Input: part model. Units: mm. Frame: model coordinates. Face numbers are marked on the shaded views. Round coordinates to 2 decimals unless told otherwise and drop trailing zeros. Loops run counter-clockwise (first coordinate to the right, second up) from the corner with the lowest first, then second, coordinate; pieces in that order, holes last.
1) Section B-B, the plane x = -1.6. Return loops of the section in (y, z), and give its area (3 significant figures).
2) Draft query along Z for the marked faces 1, 2, 3 and 4. Return one class per face: pulls with the +Z half, pulls with the -Z half, needs draft (parallel to the pull), parting line crosses it, or undercut.
3) First-contact query: pin 1 (1.5 mm diameter, centred on y = 26.5, z = -4.5, fed in from -X). Flat tip, straight axial feed; report the tip coordinate or a pass-through.
4) Ray query, line 1 along Z through (x, y) = (-1.45, 18.25); line 2 along Z through (x, y) = (-3.1, 18.25); line 3 along Y through (x, z) = (-4.3, -2). Return the intervals inside material, ascending.
5) Section A-A, the plane z = 0. Return loops of the section in (x, y).
6) Section C-C, the plane y = 18.25. Return loops of the section in (x, z).
7) Section D-D, the plane x = -3.4. Return loops of the section in (y, z).
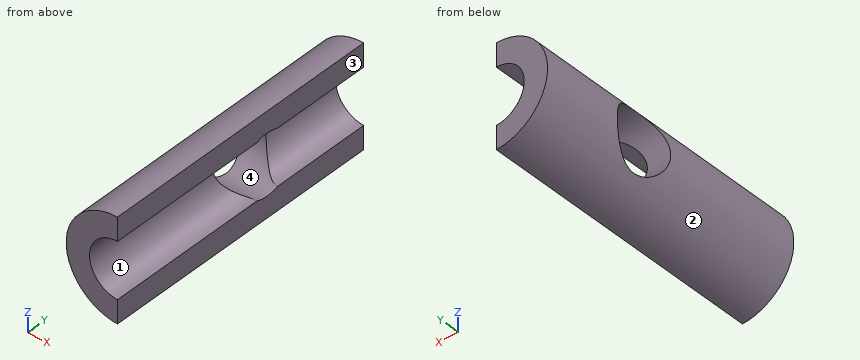
from build123d import *

# Parameters (mm, degrees)
BOSS_EXTRUDE1_DEPTH     = 30
CUT_EXTRUDE1_DEPTH      = 31.991934435
CUT_EXTRUDE1_DEPTH_BACK = 31.991934435
SKETCH2_R               = 3.25


with BuildPart() as part:
    # Sketch1 → Boss-Extrude1 (new body)
    with BuildSketch(Plane(origin=(0, 0, 0), x_dir=(1, 0, 0), z_dir=(0, 1, 0))):
        with BuildLine():
            Line((0, 5.5), (0, 3))
            ThreePointArc((0, 3), (-3, 0), (0, -3))
            Line((0, -3), (0, -5.5))
            ThreePointArc((0, -5.5), (-5.5, 0), (0, 5.5))
        make_face()
    extrude(amount=BOSS_EXTRUDE1_DEPTH)

    # Sketch2 → Cut-Extrude1 (cut, two sides: drawn at the far end of the back side and taken through both)
    with BuildSketch(Plane(origin=(0, 0, 0), x_dir=(0, 0, -1), z_dir=(1, 0, 0)).offset(-CUT_EXTRUDE1_DEPTH_BACK)):
        with Locations(Location((0, 18.25, 0), (0, 0, 337.380135052))):
            Circle(SKETCH2_R)
    extrude(amount=CUT_EXTRUDE1_DEPTH + CUT_EXTRUDE1_DEPTH_BACK, mode=Mode.SUBTRACT)


solid = part.part
Final values:
1. outline: (0, -5.26) - (30, -5.26) - (30, -2.54) - (20.28, -2.54) arc R3.25 cw to (16.22, -2.54) - (0, -2.54) - close; (0, 2.54) - (16.22, 2.54) arc R3.25 cw to (20.28, 2.54) - (30, 2.54) - (30, 5.26) - (0, 5.26) - close
1. area: 160 mm2
2. face 1: undercut
2. face 2: parting line crosses it
2. face 3: needs draft
2. face 4: undercut
3. pin 1: stops at x = -4.02
4. line 1: z = -5.31 to -3.25, 3.25 to 5.31
4. line 2: z = -4.54 to -3.25, 3.25 to 4.54
4. line 3: y = 0 to 15.69, 20.81 to 30
5. outline: (-5.5, 0) - (-3, 0) - (-3, 15) - (-5.5, 15) - close; (-5.5, 21.5) - (-3, 21.5) - (-3, 30) - (-5.5, 30) - close
6. outline: (-4.44, -3.25) arc R5.5 ccw to (0, -5.5) - (0, -3.25) - close; (-4.44, 3.25) - (0, 3.25) - (0, 5.5) arc R5.5 ccw to start
7. outline: (0, -4.32) - (30, -4.32) - (30, 4.32) - (0, 4.32) - close; hole circle Ø6.5 at (18.25, 0)
